```python
from build123d import *

# Parameters (mm, degrees)
BOSS_EXTRUDE1_DEPTH = 37
SKETCH3_R           = 11
SKETCH3_R_2         = 2
SKETCH3_R_3         = 4
CUT_EXTRUDE1_DEPTH  = 92
CUT_EXTRUDE5_DEPTH  = 35


with BuildPart() as part:
    # Sketch1 → Boss-Extrude1 (new body)
    with BuildSketch(Plane(origin=(0, 0, 0), x_dir=(1, 0, 0), z_dir=(0, 1, 0))):
        with BuildLine():
            Line((30.91362152, -11.506988518), (61.410209359, 36.471719739))
            ThreePointArc((61.410209359, 36.471719739), (65.035248289, 39.872184028), (69.84963689, 41.10738726))
            Line((69.84963689, 41.10738726), (230.684249594, 41.10738726))
            ThreePointArc((230.684249594, 41.10738726), (235.498638195, 39.872184028), (239.123677125, 36.471719739))
            Line((239.123677125, 36.471719739), (269.620264964, -11.506988518))
            ThreePointArc((269.620264964, -11.506988518), (270.941569742, -19.045741561), (266.545169913, -25.310748528))
            Line((266.545169913, -25.310748528), (256.707586966, -31.563787081))
            ThreePointArc((256.707586966, -31.563787081), (249.168833923, -32.885091859), (242.903826956, -28.488692029))
            Line((242.903826956, -28.488692029), (219.802518103, 7.855405338))
            ThreePointArc((219.802518103, 7.855405338), (216.177479173, 11.255869627), (211.363090572, 12.491072858))
            Line((211.363090572, 12.491072858), (89.170795912, 12.491072858))
            ThreePointArc((89.170795912, 12.491072858), (84.356407311, 11.255869627), (80.731368381, 7.855405338))
            Line((80.731368381, 7.855405338), (57.630059528, -28.488692029))
            Line((57.630059528, -28.488692029), (52.265727049, -36.92811956))
            Line((52.265727049, -36.92811956), (25.54928904, -19.946416049))
            Line((25.54928904, -19.946416049), (30.91362152, -11.506988518))
        make_face()
    extrude(amount=BOSS_EXTRUDE1_DEPTH)

    # Sketch3 → Cut-Extrude1 (cut)
    with BuildSketch(Plane(origin=(0, 37, 0), x_dir=(1, 0, 0), z_dir=(0, 1, 0))):
        with Locations((45.34470702, -18.309954767)):
            Circle(SKETCH3_R)
        with Locations((40.621019343, -5.235675639)):
            Circle(SKETCH3_R_2)
        with Locations((59.187759911, -17.037207093)):
            Circle(SKETCH3_R_2)
        with Locations((255.189179464, -18.309954767)):
            Circle(SKETCH3_R_3)
        with Locations((50.068394696, -31.384233896)):
            Circle(SKETCH3_R_2)
        with Locations((31.501654128, -19.582702442)):
            Circle(SKETCH3_R_2)
    extrude(amount=-CUT_EXTRUDE1_DEPTH, mode=Mode.SUBTRACT)

    # Sketch9 → Cut-Extrude5 (cut)
    with BuildSketch(Plane.XZ):
        Polygon((26.248657405, 21.639699706), (55.167500935, -23.851457954), (78.921967938, -9.666420768), (51.214594578, 37.510608863), align=None)
    extrude(amount=-CUT_EXTRUDE5_DEPTH, mode=Mode.SUBTRACT)


solid = part.part
```
For this review, take the finished solid that the model builds, in its own axes (mm). A direction names the side the tool comes from. Round coordinates to 2 decimals unless told otherwise and drop trailing zeros. Loops run counter-clockwise (first coordinate to the right, second up) from the corner with the lowest first, then second, coordinate; pieces in that order, holes last.
(1) We need section B-B (y = 18). Give the boundary of the cut face in (x, z), plus the area to 3 significant figures.
Returned:
outline: (25.55, 19.95) - (61.41, -36.47) arc R10 ccw to (69.85, -41.11) - (230.68, -41.11) arc R10 ccw to (239.12, -36.47) - (269.62, 11.51) arc R10 ccw to (266.55, 25.31) - (256.71, 31.56) arc R10 ccw to (242.9, 28.49) - (219.8, -7.86) arc R10 cw to (211.36, -12.49) - (89.17, -12.49) arc R10 cw to (80.73, -7.86) - (52.27, 36.93) - (51.75, 36.6) - (78.92, -9.67) - (55.17, -23.85) - (26.81, 20.75) - close; hole circle Ø8 at (255.19, 18.31)
area: 6,890 mm2
(2) We need section A-A (z = -2.5). Give the boundary of the cut face in (x, y), plus the area to 3 significant figures.
Returned:
outline: (39.82, 0) - (41.59, 0) - (41.59, 35) - (74.71, 35) - (74.71, 0) - (77.33, 0) - (77.33, 37) - (39.82, 37) - close; (223.21, 0) - (260.72, 0) - (260.72, 37) - (223.21, 37) - close
area: 1,620 mm2
(3) Wall thickness on line 1 along X through (y, z) = (9, -11); line 2 along X through (y, z) = (10, -4); line 3 along Z through (x, y) = (196.5, 34.5): over which ranges is each line inside the solid? List them lowest first.
Returned:
line 1: x = 45.22 to 47, 76.69 to 83.92, 216.62 to 255.31
line 2: x = 40.77 to 42.55, 75.59 to 78.28, 222.25 to 259.76
line 3: z = -41.11 to -12.49
(4) We need section D-D (x = 203). Give the boundary of the cut face in (y, z).
Returned:
outline: (0, -41.11) - (37, -41.11) - (37, -12.49) - (0, -12.49) - close
(5) Tool access review of faces 4 (the flat face through (254.158, 18.241, -12.818)), 5 (the cylindrical face through (84.42, 18.24, -11.29)), 6 (the flat face through (66.878, 17.255, -16.858)): name each direction out of +Z, -Z, +X, -X, +Y, -Y from which nothing blocks a thin tool from reaching the whole face with its end or side.
Returned:
face 4: -Z, +X, +Y, -Y
face 5: +Z, +Y, -Y
face 6: -Y
(6) We need section C-C (z = -20.5). Give the boundary of the cut face in (x, y), plus the area to 3 significant figures.
Returned:
outline: (51.26, 0) - (53.04, 0) - (53.04, 35) - (60.78, 35) - (60.78, 0) - (249.28, 0) - (249.28, 37) - (51.26, 37) - close
area: 7,060 mm2
(7) Clearance check with flat-ended pins moving along their axes: P1, Ø2.5, axis at x = 31.5, z = 19.58, coming from the +Y side; P2, Ø12, axis at x = 94.5, z = -27, coming from the -Y side; P3, Ø3, axis at y = 22.5, z = 6, coming from the -X side; P4, Ø3, axis at y = 11, z = -31, coming from the +X side. State where each tip first meets the part, or that it passes through.
Returned:
P1: passes through
P2: stops at y = 0
P3: stops at x = 33.46
P4: stops at x = 243.56
(8) Mouldability with a two-part tool opening along X and no side actions: class faces 1 (the flat face through (261.7, 18.24, 28.39)), 2 (the cylindrical face through (48.07, 36.01, 31.3)), 3 (the flat face through (38.97, 36.228, 28.477)) as released by +X, released by -X, zero draft, split by the parting line, or undercut.
Returned:
face 1: released by +X
face 2: undercut
face 3: released by -X
